Source: three-view drawing plus pictorial views. Frame: mm from the lowest corner of the part. Give positions to 0.01 mm unless a question says otherwise; leave off trailing zeros. Loops run counter-clockwise (first coordinate to the right, second up) from the corner with the lowest first, then second, coordinate; pieces in that order, holes last.
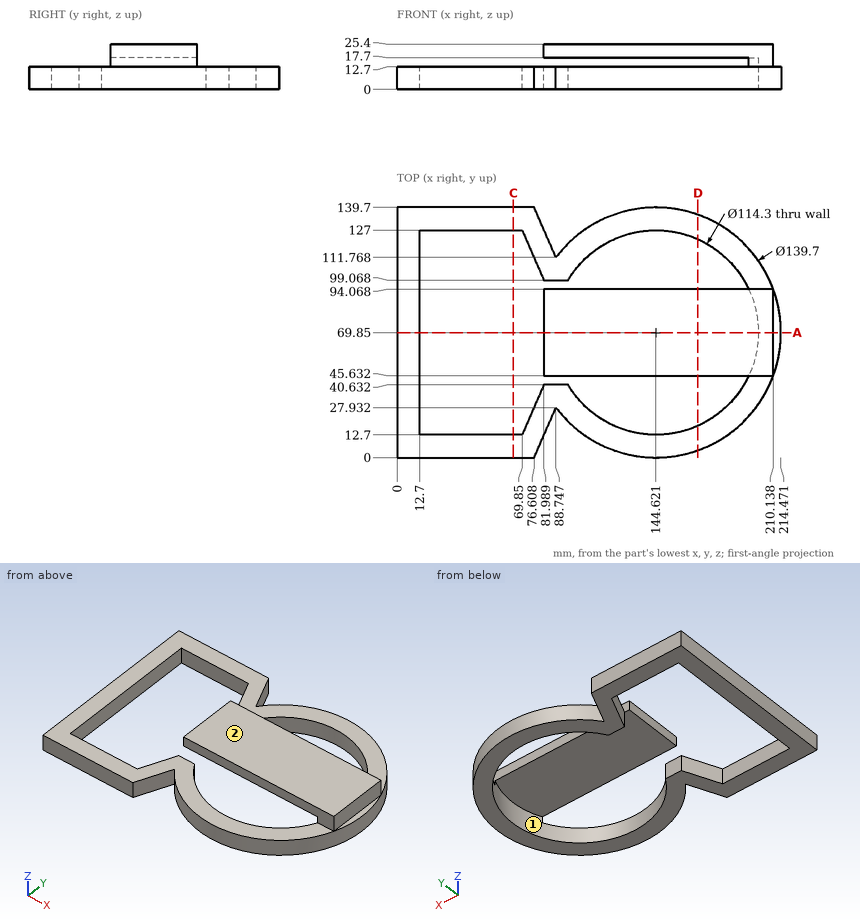
1) Ray query, probe 1 along Y at (x, z) = (30, 8.75); probe 2 along Z at (x, y) = (113.5, 130); probe 3 along X at (y, z) = (46, 21.25). Return the intervals inside material, ascending.
Checks:
probe 1: y = 0 to 12.7, 127 to 139.7
probe 2: z = 0 to 12.7
probe 3: x = 81.99 to 210.14
2) Cut plane A-A (y = 69.85). Return loops of the section in (x, z).
Checks:
outline: (0, 0) - (12.7, 0) - (12.7, 12.7) - (0, 12.7) - close; (81.99, 17.7) - (201.77, 17.7) - (201.77, 0) - (214.47, 0) - (214.47, 12.7) - (210.14, 12.7) - (210.14, 25.4) - (81.99, 25.4) - close
3) Cut plane C-C (x = 65). Return loops of the section in (y, z).
Checks:
outline: (0, 0) - (12.7, 0) - (12.7, 12.7) - (0, 12.7) - close; (127, 0) - (139.7, 0) - (139.7, 12.7) - (127, 12.7) - close
4) Cut plane D-D (x = 168). Return loops of the section in (y, z).
Checks:
outline: (4.03, 0) - (17.7, 0) - (17.7, 12.7) - (4.03, 12.7) - close; (45.63, 17.7) - (94.07, 17.7) - (94.07, 25.4) - (45.63, 25.4) - close; (122, 0) - (135.67, 0) - (135.67, 12.7) - (122, 12.7) - close
5) Pull-direction query (X, two-part tool) for the marked faces 1 and 2; classes: released by +X, released by -X, zero draft, split by the parting line, or undercut.
Checks:
face 1: undercut
face 2: zero draft
6) Contact query for flat-ended pins moving along their axis: P1, Ø4, axis at x = 87, z = 9.5, coming from the -Y side (1 decimal); P2, Ø24, axis at x = 116.5, y = 78.5, coming from the -Z side; P3, Ø10, axis at y = 87, z = 4.5, coming from the +X side; P4, Ø10, axis at y = 119, z = 9.5, coming from the -X side. Output: stop coordinate, or through.
Checks:
P1: stops at y = 19.3
P2: stops at z = 17.7
P3: stops at x = 213.41
P4: stops at x = 0
